```python
from build123d import *

# Parameters (mm, degrees)
SKETCH1_W           = 90
SKETCH1_H           = 25
BOSS_EXTRUDE1_DEPTH = 25.05
FILLET1_R           = 12.5
SKETCH2_R           = 1.5
CUT_EXTRUDE1_DEPTH  = 5


with BuildPart() as part:
    # Sketch1 → Boss-Extrude1 (new body)
    with BuildSketch(Plane(origin=(0, 0, 0), x_dir=(1, 0, 0), z_dir=(0, 1, 0))):
        with Locations((45, 12.5)):
            Rectangle(SKETCH1_W, SKETCH1_H)
    extrude(amount=BOSS_EXTRUDE1_DEPTH)

    # Fillet1
    fillet1_edges = [part.edges().sort_by_distance(p)[0] for p in [
        (90, 12.525, 0),
        (90, 12.525, -25),
        (0, 12.525, 0),
        (0, 12.525, -25),
    ]]
    fillet(fillet1_edges, radius=FILLET1_R - 0.0001)  # a hair under: the kernel refuses the full size

    # Sketch2 → Cut-Extrude1 (cut)
    with BuildSketch(Plane.XZ):
        with Locations(Location((22.5, -12.5, 0), (0, 0, 270))):
            Circle(SKETCH2_R)
        with Locations(Location((67.5, -12.5, 0), (0, 0, 270))):
            Circle(SKETCH2_R)
    extrude(amount=-CUT_EXTRUDE1_DEPTH, mode=Mode.SUBTRACT)


solid = part.part
```
Verification items for the finished model (mm, model axes). A direction names the side the tool comes from. Round coordinates to 2 decimals unless told otherwise and drop trailing zeros. Loops run counter-clockwise (first coordinate to the right, second up) from the corner with the lowest first, then second, coordinate; pieces in that order, holes last. Notation, with made-up numbers: (1, 63) -> (31, 63) arc R33 cw to (31, 95) -> close; hole circle Ø1 at (-20, 47). An arc over 180 degrees is marked (long way). Answer as a JSON object with one key per item and string values.
Q1. Section check C-C (z = -5.25). Record the boundary of the cut face in (x, y), then the cut area to 3 significant figures.
Data:
{"outline": "(2.32, 0) -> (87.68, 0) -> (87.68, 25.05) -> (2.32, 25.05) -> close", "area": "2,140 mm2"}
Q2. Draft check along X on faces 3 (the cylindrical face through (86.436, 12.7, -21.241)), 4 (the flat face through (45, 12, -25)), 5 (the flat face through (68, 5, -12)), 6 (the cylindrical face through (3.564, 12.7, -21.241)). Enter one of: pulls with the +X half, pulls with the -X half, needs draft (parallel to the pull), parting line crosses it, or undercut.
Data:
{"face 3": "pulls with the +X half", "face 4": "needs draft", "face 5": "undercut", "face 6": "pulls with the -X half"}
Q3. Scan lines: line 1 (X direction, y = 2, z = -12.5); line 2 (Z direction, x = 67.5, y = 3.8); line 3 (X direction, y = 7.5, z = -12). Record each from-to range of solid material in increasing order. Write a range as from..to.
Data:
{"line 1": "x = 0..21, 24..66, 69..90", "line 2": "z = -25..-14, -11..0", "line 3": "x = 0.01..89.99"}
Q4. Access from +Z, -Z, +X, -X, +Y, -Y to the whole of each face (thin tool, end or side, straight path). Record for faces 1 (the cylindrical face through (3.564, 12.7, -3.759)), 2 (the cylindrical face through (68.765, 2.465, -13.306)).
Data:
{"face 1": "+Z, -X, +Y, -Y", "face 2": "-Y"}
Q5. Section check D-D (x = 6.5). Record the boundary of the cut face in (y, z), then the cut area to 3 significant figures.
Data:
{"outline": "(0, -23.47) -> (25.05, -23.47) -> (25.05, -1.53) -> (0, -1.53) -> close", "area": "549 mm2"}
Q6. Go/stop test with flat-tipped pins: P1, Ø5, axis at y = 11.5, z = -3, coming from the -X side; P2, Ø8, axis at y = 6.5, z = -3.5, coming from the -X side; P3, Ø0.9, axis at x = 68, z = -12, coming from the -Y side. Record where each tip stops, or that it passes through.
Data:
{"P1": "stops at x = 2.14", "P2": "stops at x = 1.04", "P3": "stops at y = 5"}
Q7. Section check B-B (x = 67.5). Record the boundary of the cut face in (y, z).
Data:
{"outline": "(0, -25) -> (25.05, -25) -> (25.05, 0) -> (0, 0) -> (0, -11) -> (5, -11) -> (5, -14) -> (0, -14) -> close"}
